Part print with two shaded views. Sizes in mm from the minimum x, y, z corner. A direction names the side the tool comes from. Round coordinates to 2 decimals unless told otherwise and drop trailing zeros. Order: outer loops, then holes, each group sorted by start corner. A loop starts at its lowest first (then second) coordinate and runs counter-clockwise, first axis right, second up. Notation, with made-up numbers: (-10.75, -38) -> (7.25, -38) arc R14 ccw to (7.25, -32) -> close; hole circle Ø8 at (-21, 74.25). An arc over 180 degrees is marked (long way). Put each result on its own line as item: value. Start each with the question number.
Q1. Flat gauge pins, fed straight in: P1, Ø12, axis at x = 10.5, z = 45.5, coming from the -Y side; P2, Ø1.5, axis at x = 20, z = 41, coming from the +Y side; P3, Ø8, axis at x = 21.5, y = 180, coming from the +Z side; P4, Ø14, axis at x = 10.5, z = 55.5, coming from the +Y side. Where does each tip first touch, or does it go through?
Q2. 3-axis set-ups, long thin cutter, end or side, ignore diameter. For the marked faces 1 and 2: which of +Z, -Z, +X, -X, +Y, -Y reach the whole face in a straight line?
Q3. Cut at C-C, the plane x = 14. List the corners of the cut face in (y, z), and give its area (3 significant figures).
Q4. Cut at D-D, the plane z = 60. List the corners of the cut face in (x, y).
Q5. Probe L1, parallel to Z at x = 9, y = 153.5; L2, parallel to X at y = 171.5, z = 29; L3, parallel to Z at x = 12, y = 77.5. List the from-to ranges inside material, lowest first.
Q6. Cut at B-B, the plane z = 30.5. List the corners of the cut face in (x, y).
Q7. Pull direction X, two halves, no side cores. Call the marked faces 3, 4 and 5: released by +X, released by -X, zero draft, split by the parting line, or undercut.
Q8. Cut at A-A, the plane y = 153.5. List the corners of the cut face in (x, z), and give its area (3 significant figures).
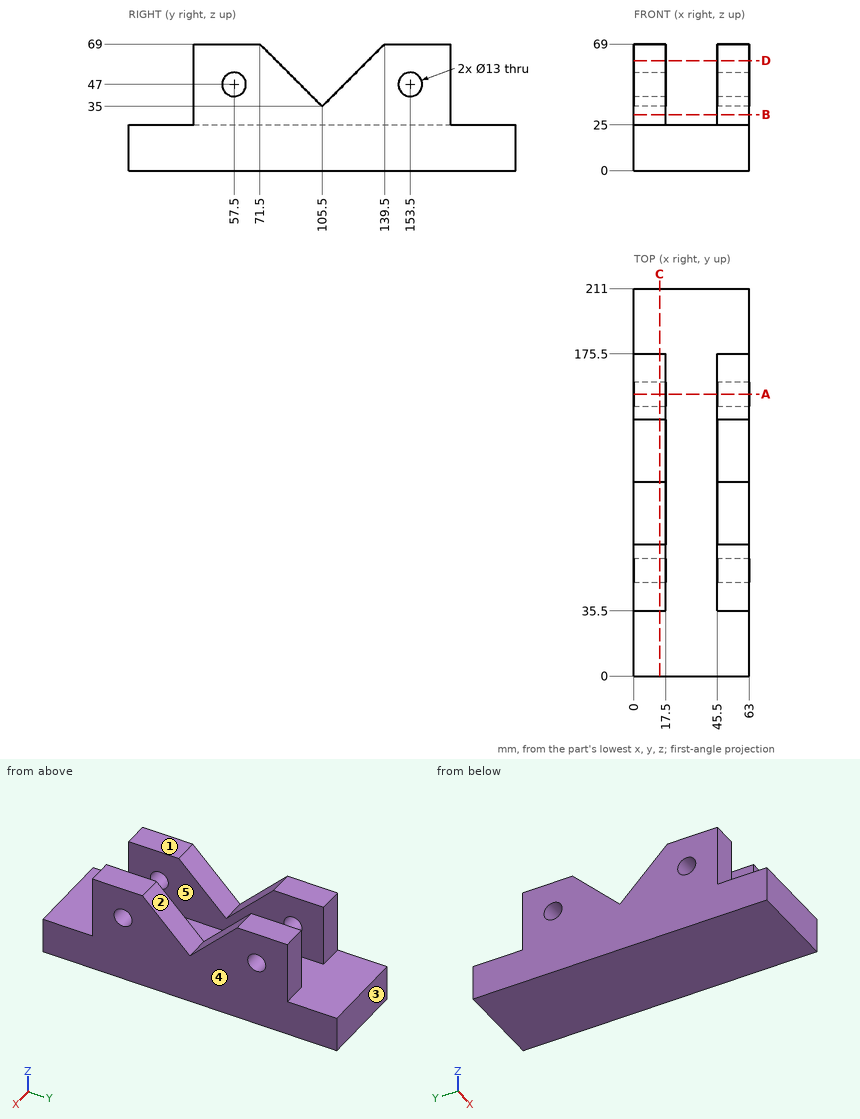
Ans:
1. P1: stops at y = 35.5
1. P2: passes through
1. P3: stops at z = 25
1. P4: stops at y = 175.5
2. face 1: +Z, +X, -X, +Y, -Y
2. face 2: +Z, +X, -X
3. outline: (0, 0) -> (211, 0) -> (211, 25) -> (175.5, 25) -> (175.5, 69) -> (139.5, 69) -> (105.5, 35) -> (71.5, 69) -> (35.5, 69) -> (35.5, 25) -> (0, 25) -> close; hole circle Ø13 at (57.5, 47); hole circle Ø13 at (153.5, 47)
3. area: 10,000 mm^2
4. outline: (0, 35.5) -> (17.5, 35.5) -> (17.5, 80.5) -> (0, 80.5) -> close; (0, 130.5) -> (17.5, 130.5) -> (17.5, 175.5) -> (0, 175.5) -> close; (45.5, 35.5) -> (63, 35.5) -> (63, 80.5) -> (45.5, 80.5) -> close; (45.5, 130.5) -> (63, 130.5) -> (63, 175.5) -> (45.5, 175.5) -> close
5. L1: z = 0 to 40.5, 53.5 to 69
5. L2: x = 0 to 17.5, 45.5 to 63
5. L3: z = 0 to 63
6. outline: (0, 35.5) -> (17.5, 35.5) -> (17.5, 175.5) -> (0, 175.5) -> close; (45.5, 35.5) -> (63, 35.5) -> (63, 175.5) -> (45.5, 175.5) -> close
7. face 3: zero draft
7. face 4: released by +X
7. face 5: undercut
8. outline: (0, 0) -> (63, 0) -> (63, 40.5) -> (45.5, 40.5) -> (45.5, 25) -> (17.5, 25) -> (17.5, 40.5) -> (0, 40.5) -> close; (0, 53.5) -> (17.5, 53.5) -> (17.5, 69) -> (0, 69) -> close; (45.5, 53.5) -> (63, 53.5) -> (63, 69) -> (45.5, 69) -> close
8. area: 2,660 mm^2
